```python
from build123d import *

# Parameters (mm, degrees)
IZIM1_W                                 = 40.658634346
IZIM1_H                                 = 22.072921898
Y_KSEKLIK_EKSTR_ZYON3_DEPTH             = 1.5
IZIM10_W                                = 40.658634346
IZIM10_H                                = 22.072921898
Y_KSEKLIK_EKSTR_ZYON5_DEPTH             = 1.5
Y_KSEKLIK_EKSTR_ZYON6_DEPTH             = 1.5
IZIM12_W                                = 40.658634346
IZIM12_H                                = 22.072921898
KES_EKSTR_ZYON1_DEPTH                   = 5
KES_EKSTR_ZYON1_DEPTH_BACK              = 3
RADYUS1_R                               = 3
Y_KSEKLIK_EKSTR_ZYON7_REACH             = 3.5
Y_KSEKLIK_EKSTR_ZYON7_DIRECTION_2_REACH = 31.45
IZIM18_R                                = 0.6
KES_EKSTR_ZYON3_DEPTH                   = 7
KES_EKSTR_ZYON3_DEPTH_BACK              = 3
SKETCH1_R                               = 1
CUT_EXTRUDE1_DEPTH                      = 3


with BuildPart() as part:
    # Çizim1 → Yükseklik-Ekstrüzyon3 (new body)
    with BuildSketch(Plane(origin=(0, 0, 0), x_dir=(1, 0, 0), z_dir=(0, 1, 0))):
        with Locations((1.2, 0)):
            Rectangle(IZIM1_W, IZIM1_H)
        with BuildLine():
            Line((1.9, -6.45), (1.9, -3.295349698))
            Line((1.9, -3.295349698), (16.626291793, -1.99221515))
            ThreePointArc((16.626291793, -1.99221515), (18.45, 0), (16.626291793, 1.99221515))
            Line((16.626291793, 1.99221515), (1.9, 3.295349698))
            Line((1.9, 3.295349698), (1.9, 6.45))
            ThreePointArc((1.9, 6.45), (0, 8.35), (-1.9, 6.45))
            Line((-1.9, 6.45), (-1.9, 2.87967012))
            ThreePointArc((-1.9, 2.87967012), (-2.057742862, 2.769150468), (-2.209072203, 2.65))
            Line((-2.209072203, 2.65), (-14.159121967, 1.99702088))
            ThreePointArc((-14.159121967, 1.99702088), (-16.05, 0), (-14.159121967, -1.99702088))
            Line((-14.159121967, -1.99702088), (-2.209072203, -2.65))
            ThreePointArc((-2.209072203, -2.65), (-2.057742862, -2.769150468), (-1.9, -2.87967012))
            Line((-1.9, -2.87967012), (-1.9, -6.45))
            ThreePointArc((-1.9, -6.45), (0, -8.35), (1.9, -6.45))
        make_face(mode=Mode.SUBTRACT)
    extrude(amount=Y_KSEKLIK_EKSTR_ZYON3_DEPTH)

    # Çizim10 → Yükseklik-Ekstrüzyon5 (add)
    with BuildSketch(Plane(origin=(0, 1.5, 0), x_dir=(1, 0, 0), z_dir=(0, 1, 0))):
        with Locations((1.2, 0)):
            Rectangle(IZIM10_W, IZIM10_H)
    extrude(amount=Y_KSEKLIK_EKSTR_ZYON5_DEPTH)

    # Çizim11 → Yükseklik-Ekstrüzyon6 (add, symmetric)
    with BuildSketch(Plane(origin=(0, 0, 0), x_dir=(0, 0, -1), z_dir=(1, 0, 0))):
        Polygon((18.5, 10.980931434), (1.5, 10.980931434), (1.5, 1.777726909), (-1.5, 1.777726909), (-1.5, 10.980931434), (-1.5, 13.980931434), (1.5, 13.980931434), (21.5, 13.980931434), (21.5, -24.019068566), (18.5, -24.019068566), align=None)
    extrude(amount=Y_KSEKLIK_EKSTR_ZYON6_DEPTH, both=True)

    # Çizim12 → Kes-Ekstrüzyon1 (cut, two sides)
    with BuildSketch(Plane(origin=(0, 0, 0), x_dir=(1, 0, 0), z_dir=(0, 1, 0))) as kes_ekstr_zyon1_sk:
        with Locations((1.2, 0)):
            Rectangle(IZIM12_W, IZIM12_H)
        Polygon((0, -9.45), (-17.05, -9.45), (-17.05, 9.45), (19.45, 9.45), (19.45, -9.45), align=None, mode=Mode.SUBTRACT)
    extrude(amount=KES_EKSTR_ZYON1_DEPTH, mode=Mode.SUBTRACT)
    extrude(kes_ekstr_zyon1_sk.sketch, amount=-KES_EKSTR_ZYON1_DEPTH_BACK, mode=Mode.SUBTRACT)

    # Radyus1
    radyus1_edges = [part.edges().sort_by_distance(p)[0] for p in [
        (-1.5, 3, 0),
        (0, 3, -1.5),
        (0, 3, 1.5),
        (1.5, 3, 0),
        (0, 13.980931434, -21.5),
        (0, 13.980931434, 1.5),
        (0, 10.980931434, -1.5),
        (0, 10.980931434, -18.5),
    ]]
    fillet(radyus1_edges, radius=RADYUS1_R)

    # Yükseklik-Ekstrüzyon7: up to this face of the body (flat: up to its plane)
    y_kseklik_ekstr_zyon7_end = Plane(part.part.faces().sort_by_distance((0, -6.519068566, -21.5))[0])
    # Çizim13 → Yükseklik-Ekstrüzyon7 (add, up to the picked face)
    with BuildSketch(Plane(origin=(0, 0, -20), x_dir=(-1, 0, 0), z_dir=(0, 0, -1)), mode=Mode.PRIVATE) as y_kseklik_ekstr_zyon7_sk1:
        Polygon((-26.108304445, 2.483027661), (-26.108304445, -23.516972339), (0.891695555, -23.516972339), (0.891695555, -2.497903773), (0.891695555, 2.483027661), align=None)
    y_kseklik_ekstr_zyon7_tool1 = split(extrude(y_kseklik_ekstr_zyon7_sk1.sketch, amount=Y_KSEKLIK_EKSTR_ZYON7_REACH, mode=Mode.PRIVATE), bisect_by=y_kseklik_ekstr_zyon7_end, keep=Keep.BOTH, mode=Mode.PRIVATE)
    add(y_kseklik_ekstr_zyon7_tool1.solids().sort_by_distance((12.608304, -10.516972, -20))[0])

    # Yükseklik-Ekstrüzyon7 direction 2: up to this face of the body (flat: up to its plane)
    y_kseklik_ekstr_zyon7_direction_2_end = Plane(part.part.faces().sort_by_distance((0, -8.019068566, -18.5))[0])
    # Çizim13 → Yükseklik-Ekstrüzyon7 direction 2 (add, up to the picked face)
    with BuildSketch(Plane(origin=(0, 0, -20), x_dir=(-1, 0, 0), z_dir=(0, 0, -1)), mode=Mode.PRIVATE) as y_kseklik_ekstr_zyon7_direction_2_sk1:
        Polygon((-26.108304445, 2.483027661), (-26.108304445, -23.516972339), (0.891695555, -23.516972339), (0.891695555, -2.497903773), (0.891695555, 2.483027661), align=None)
    y_kseklik_ekstr_zyon7_direction_2_tool1 = split(extrude(y_kseklik_ekstr_zyon7_direction_2_sk1.sketch, amount=-Y_KSEKLIK_EKSTR_ZYON7_DIRECTION_2_REACH, mode=Mode.PRIVATE), bisect_by=y_kseklik_ekstr_zyon7_direction_2_end, keep=Keep.BOTH, mode=Mode.PRIVATE)
    add(y_kseklik_ekstr_zyon7_direction_2_tool1.solids().sort_by_distance((12.608304, -10.516972, -20))[0])

    # Çizim18 → Kes-Ekstrüzyon3 (cut, two sides)
    with BuildSketch(Plane.XZ.offset(-1.5)) as kes_ekstr_zyon3_sk:
        with Locations((-14.45, 0)):
            Circle(IZIM18_R)
        with Locations((16.85, 0)):
            Circle(IZIM18_R)
    extrude(amount=KES_EKSTR_ZYON3_DEPTH, mode=Mode.SUBTRACT)
    extrude(kes_ekstr_zyon3_sk.sketch, amount=-KES_EKSTR_ZYON3_DEPTH_BACK, mode=Mode.SUBTRACT)

    # Sketch1 → Cut-Extrude1 (cut)
    with BuildSketch(Plane(origin=(0, 0, -21.5), x_dir=(-1, 0, 0), z_dir=(0, 0, -1))):
        with Locations((-2.999001891, -0.516972339)):
            Circle(SKETCH1_R)
        with Locations((-2.999001891, -21.516972339)):
            Circle(SKETCH1_R)
        with Locations((-15.499001891, -21.516972339)):
            Circle(SKETCH1_R)
        with Locations((-15.499001891, -0.516972339)):
            Circle(SKETCH1_R)
    extrude(amount=-CUT_EXTRUDE1_DEPTH, mode=Mode.SUBTRACT)


solid = part.part
```
For this review, take the finished solid that the model builds, in its own axes (mm). A direction names the side the tool comes from. Coordinates: 2 decimals unless noted, no trailing zeros. Write each loop counter-clockwise with the first axis right and the second up, starting at its lowest first coordinate (ties: lowest second). Pieces come first, ordered by that corner, then holes. Notation, with made-up numbers: (4, 59.5) - (42, 59.5) arc R18 ccw to (42, 94.5) - close; hole circle Ø8 at (59.25, 79). An arc over 180 degrees is marked (long way). Put each result on its own line as item: value.
1. Mouldability with a two-part tool opening along Z and no side actions: class faces 5 (the cylindrical face through (-0.021, 13.079, -20.645)), 6 (the cylindrical face through (-0.021, 13.125, 0.598)), 7 (the flat face through (1.5, 12, -10)), 8 (the flat face through (-8.1, 0.74, -2.33)) as released by +Z, released by -Z, zero draft, split by the parting line, or undercut.
Values found:
face 5: released by -Z
face 6: released by +Z
face 7: zero draft
face 8: undercut
2. Machinability: for faces 1 (the flat face through (14, 2.483, -20)), 2 (the flat face through (0, 10.981, -10)), 3 (the cylindrical face through (-16.05, 0.74, -0.04)), 4 (the flat face through (14, -23.517, -20)), which of the approach directions +Z, -Z, +X, -X, +Y, -Y give a long, thin tool a straight path to every point of the face, cutting with its end or side? Answer none if there is none.
Values found:
face 1: -Z, +X, +Y
face 2: +X, -X
face 3: -Y
face 4: +Z, -Z, +X, -Y
3. Add section B-B, the plane z = 0. Give the boundary of the cut face in (x, y), then the cut area to 4 significant figures.
Values found:
outline: (-17.05, 0) - (-16.05, 0) - (-16.05, 1.5) - (-15.05, 1.5) - (-15.05, 3) - (-17.05, 3) - close; (-13.85, 1.5) - (16.25, 1.5) - (16.25, 3) - (4.5, 3) arc R3 cw to (1.5, 6) - (1.5, 13.58) - (-1.5, 13.58) - (-1.5, 6) arc R3 cw to (-4.5, 3) - (-13.85, 3) - close; (17.45, 1.5) - (18.45, 1.5) - (18.45, 0) - (19.45, 0) - (19.45, 3) - (17.45, 3) - close
area: 89.75 mm²
4. Wall thickness on probe 1 along Z at (x, y) = (16, 2); probe 2 along Z at (x, y) = (16, -7.5); probe 3 along Y at (x, z) = (-8.5, -5.5): over which ranges is each line inside the solid? List them lowest first.
Values found:
probe 1: -21.5 to -18.5, -9.45 to 9.45
probe 2: -21.5 to -18.5
probe 3: 0 to 3
5. For pin 1 (1 mm diameter, centred on x = -0.5, y = 9, fed in from +Z); pin 2 (13.5 mm diameter, centred on x = 5, z = -2, fed in from -Y); pin 3 (1.4 mm diameter, centred on x = 16.85, z = 0, fed in from +Y); pin 4 (9.5 mm diameter, centred on x = -0.5, z = 2, fed in from +Y), all flat-tipped, find the tip position at first contact; note any pin that passes through.
Values found:
pin 1: z = 1.5
pin 2: y = 0
pin 3: y = 3
pin 4: y = 13.98
6. Add section A-A, the plane x = 0. Give the boundary of the cut face in (y, z).
Values found:
outline: (-24.02, -21.5) - (10.98, -21.5) arc R3 ccw to (13.98, -18.5) - (13.98, -1.5) arc R3 ccw to (10.98, 1.5) - (6, 1.5) arc R3 cw to (3, 4.5) - (3, 9.45) - (0, 9.45) - (0, 8.35) - (1.5, 8.35) - (1.5, -8.35) - (0, -8.35) - (0, -9.45) - (3, -9.45) - (3, -4.5) arc R3 cw to (6, -1.5) - (7.98, -1.5) arc R3 cw to (10.98, -4.5) - (10.98, -15.5) arc R3 cw to (7.98, -18.5) - (-24.02, -18.5) - close
7. Add section C-C, the plane y = -14. Give the boundary of the cut face in (x, z), then the cut area to 3 significant figures.
Values found:
outline: (-1.5, -21.5) - (26.11, -21.5) - (26.11, -18.5) - (-1.5, -18.5) - close
area: 82.8 mm²
8. Add section D-D, the plane x = -10. Give the boundary of the cut face in (y, z).
Values found:
outline: (0, -9.45) - (3, -9.45) - (3, 9.45) - (0, 9.45) - (0, 2.22) - (1.5, 2.22) - (1.5, -2.22) - (0, -2.22) - close
